Verification items for this drawing (mm, ordinates from the low corner). Give positions to 0.01 mm unless a question says otherwise; leave off trailing zeros. Order: outer loops, then holes, each group sorted by start corner. A loop starts at its lowest first (then second) coordinate and runs counter-clockwise, first axis right, second up. Notation, with made-up numbers: M 51.25,77.5 L 84.25,77.5 A15 cw 84.25,81.5 Z; hole C 65.25,-24 d8. An arc over 180 degrees is marked long. Return JSON: item names as keys, results as strings. Group by question number.
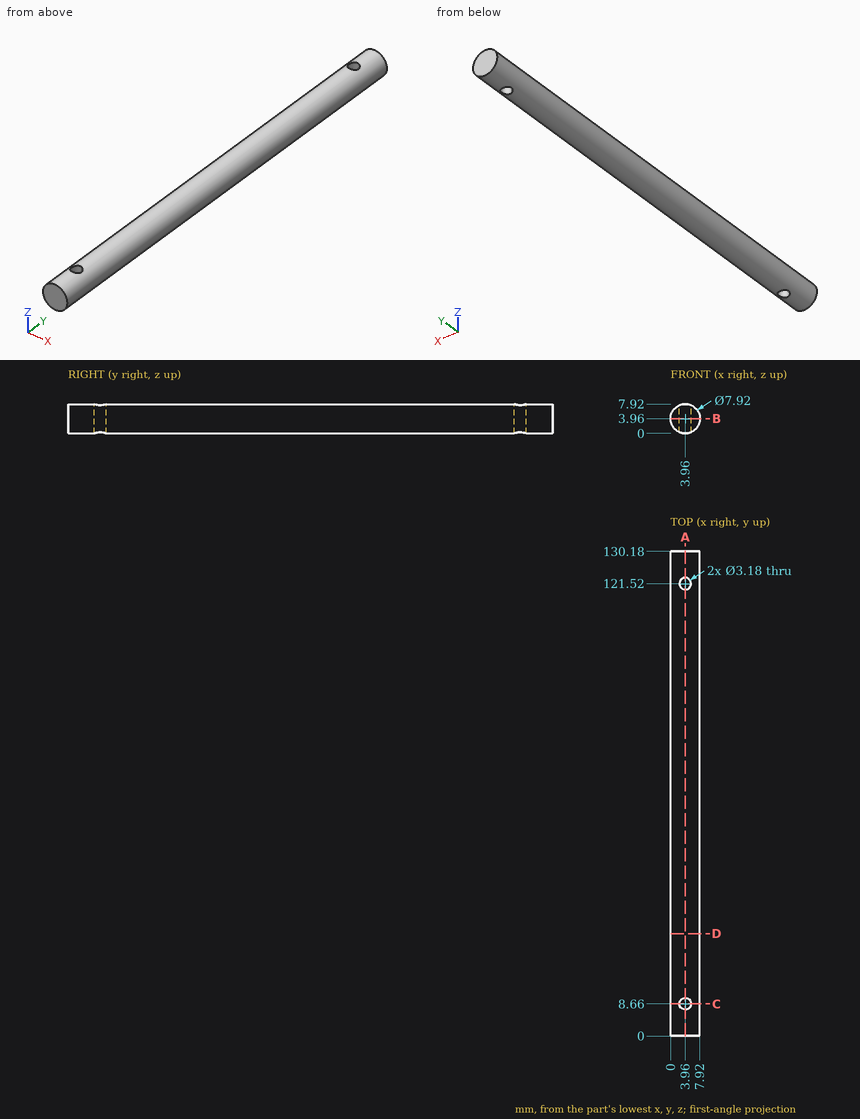
1) Sectioned sample at B-B on z = 3.96. Record the boundary of the cut face in (x, y).
2) Material ranges on line 1 along Y through (x, z) = (3.5, 3.25); line 2 along Y through (x, z) = (5, 3.25); line 3 along X through (y, z) = (8.66, 2.25), recorded low to high.
3) Depth check by flat-ended pin: P1, Ø2, axis at x = 1.5, y = 113.5, coming from the -Z side; P2, Ø1.9, axis at x = 3.96, y = 8.66, coming from the +Z side; P3, Ø1, axis at x = 2.5, y = 28.5, coming from the +Z side. Enter the tip coordinate at first touch or a pass-through.
4) Sectioned sample at C-C on y = 8.66. Record the boundary of the cut face in (x, z).
5) Sectioned sample at A-A on x = 3.96. Record the boundary of the cut face in (y, z).
6) Sectioned sample at D-D on y = 27.5. Record the boundary of the cut face in (x, z).
Reply:
{
 "1": {"outline": "M 0,0 L 7.92,0 L 7.92,130.18 L 0,130.18 Z; hole C 3.96,8.66 d3.18; hole C 3.96,121.52 d3.18"},
 "2": {"line 1": "0 to 7.14, 10.18 to 120, 123.04 to 130.18", "line 2": "0 to 7.46, 9.86 to 120.32, 122.72 to 130.18", "line 3": "0.39 to 2.37, 5.55 to 7.53"},
 "3": {"P1": "z = 0.28", "P2": "through", "P3": "z = 7.8"},
 "4": {"outline": "M 2.37,0.33 L 2.37,7.59 A3.96 ccw Z; M 5.55,0.33 A3.96 ccw 5.55,7.59 Z"},
 "5": {"outline": "M 0,0 L 7.07,0 L 7.07,7.92 L 0,7.92 Z; M 10.25,0 L 119.93,0 L 119.93,7.92 L 10.25,7.92 Z; M 123.11,0 L 130.18,0 L 130.18,7.92 L 123.11,7.92 Z"},
 "6": {"outline": "C 3.96,3.96 d7.92"}
}
